from build123d import *

# Parameters (mm, degrees)
F0_W     = 900
F0_H     = 200
F0_W_2   = 200
F0_H_2   = 900
F1_DEPTH = 30
F2_SIZE  = 30
F3_SIZE  = 10


with BuildPart() as f1:
    # F0 (on Top) → F1 (new body)
    with BuildSketch(Plane.XY):
        with Locations((-1543.7867450795, 647.8599071422)):
            Rectangle(F0_W, F0_H)
        with Locations((-993.7867450795, 1197.8599071422)):
            Rectangle(F0_W_2, F0_H_2)
        with Locations((-993.7867450795, 647.8599071422)):
            Rectangle(F0_W_2, F0_H)
        with Locations((-443.7867450795, 647.8599071422)):
            Rectangle(F0_W, F0_H)
        with Locations((-993.7867450795, 97.8599071422)):
            Rectangle(F0_W_2, F0_H_2)
    extrude(amount=F1_DEPTH)

    # F2
    f2_edges = [f1.edges().sort_by_distance(p)[0] for p in [
        (-1093.786745, 747.859907, 15),
        (-1993.786745, 747.859907, 15),
        (-1993.786745, 547.859907, 15),
        (-1093.786745, 547.859907, 15),
        (-1093.786745, -352.140093, 15),
        (-893.786745, -352.140093, 15),
        (-893.786745, 547.859907, 15),
        (6.213255, 547.859907, 15),
        (6.213255, 747.859907, 15),
        (-893.786745, 747.859907, 15),
        (-893.786745, 1647.859907, 15),
        (-1093.786745, 1647.859907, 15),
    ]]
    chamfer(f2_edges, length=F2_SIZE)

    # F3
    f3_edges = [f1.edges().sort_by_distance(p)[0] for p in [
        (-993.786745, -352.140093, 30),
        (6.213255, 647.859907, 30),
        (-993.786745, 1647.859907, 30),
        (-1993.786745, 647.859907, 30),
    ]]
    chamfer(f3_edges, length=F3_SIZE)


solid = f1.part
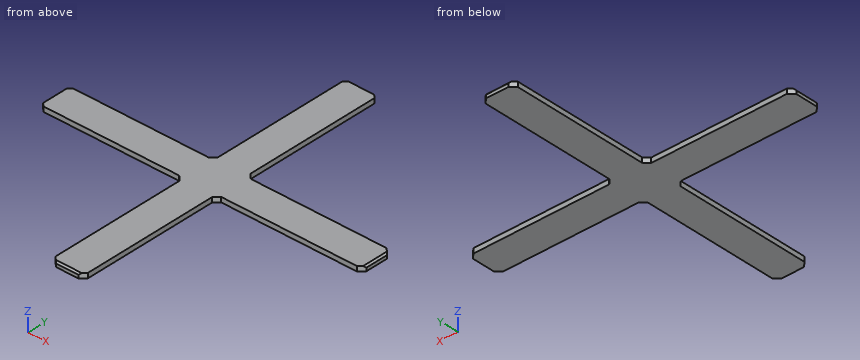
Work out the finished part from the listing and answer in its coordinate system (mm). Coordinates: 2 decimals unless noted, no trailing zeros. Write each loop counter-clockwise with the first axis right and the second up, starting at its lowest first coordinate (ties: lowest second). Pieces come first, ordered by that corner, then holes. Notation, with made-up numbers: M 4,11.5 L 61,11.5 A8 cw 61,20.5 Z; hole C 14.25,-40 d11. An arc over 180 degrees is marked long. Answer as CSV lines item,"result". Start each with the question number.
Item 1: Flat-ended cylindrical pins translate along their axes: P1, Ø5, axis at y = 1057, z = 26.5, coming from the +X side; P2, Ø1.5, axis at x = -385.5, z = 15, coming from the +Y side; P3, Ø10, axis at x = -809.5, z = 24.5, coming from the -Y side. Find the tip coordinate at first contact, or state that the pin passes through.
Item 2: Consider L1, parallel to Y at x = -1584, z = 19; L2, parallel to X at y = 189.5, z = 16.5; L3, parallel to X at y = 756, z = 28. Determine where each line is inside the solid, lowest interval first.
Item 3: Section C-C on x = -1840 is taken. Write down the section's boundary in (y, z).
Item 4: Section A-A on z = 14 is taken. Write down the section's boundary in (x, y), and give its area (3 significant figures).
Item 5: Section B-B on y = 141 is taken. Write down the section's boundary in (x, z), and give its area (3 significant figures).
Checks:
1,P1,"stops at x = -893.79"
1,P2,"stops at y = 747.86"
1,P3,"stops at y = 547.86"
2,L1,"y = 547.86 to 747.86"
2,L2,"x = -1093.79 to -893.79"
2,L3,"x = -1115.65 to -871.93"
3,outline,"M 547.86,0 L 747.86,0 L 747.86,30 L 547.86,30 Z"
4,outline,"M -1993.79,577.86 L -1963.79,547.86 L -1123.79,547.86 L -1093.79,517.86 L -1093.79,-322.14 L -1063.79,-352.14 L -923.79,-352.14 L -893.79,-322.14 L -893.79,517.86 L -863.79,547.86 L -23.79,547.86 L 6.21,577.86 L 6.21,717.86 L -23.79,747.86 L -863.79,747.86 L -893.79,777.86 L -893.79,1617.86 L -923.79,1647.86 L -1063.79,1647.86 L -1093.79,1617.86 L -1093.79,777.86 L -1123.79,747.86 L -1963.79,747.86 L -1993.79,717.86 Z"
4,area,"758,000 mm²"
5,outline,"M -1093.79,0 L -893.79,0 L -893.79,30 L -1093.79,30 Z"
5,area,"6,000 mm²"
